Read the model definition and answer for the solid it produces. Units are mm, in the model's axes. A direction names the side the tool comes from. Coordinates: 2 decimals unless noted, no trailing zeros. Write each loop counter-clockwise with the first axis right and the second up, starting at its lowest first coordinate (ties: lowest second). Pieces come first, ordered by that corner, then holes. Notation, with made-up numbers: (76, -26) -> (130, -26) arc R25 ccw to (130, -8) -> close; hole circle Ø9 at (71.25, 61). An arc over 180 degrees is marked (long way). Return JSON: item names as keys, results as strings.
Autodesk Fusion 360 part; units mm, degrees
sketch "Sketch1" plane through (0, 0, 0) normal (0, 1, 0) x (1, 0, 0)
  line L0 (0, 0) -> (41, 0)
  line L1 (41, 0) -> (41, -41)
  line L2 (41, -41) -> (0, -41)
  line L3 (0, -41) -> (0, 0)
  line L4 (0, -20.5) -> (41, -20.5) construction
  line L5 (20.5, 0) -> (20.5, -41) construction
  circle A0 centre (20.5, -20.5) radius 12.5
  line L6 (36, -36) -> (5, -36) construction
  line L7 (5, -36) -> (5, -5) construction
  line L8 (5, -5) -> (36, -5) construction
  line L9 (36, -5) -> (36, -36) construction
  line L10 (36, -36) -> (5, -5) construction
  line L11 (5, -36) -> (36, -5) construction
  circle A1 centre (5, -36) radius 1.8
  circle A2 centre (36, -36) radius 1.8
  circle A3 centre (36, -5) radius 1.8
  circle A4 centre (5, -5) radius 1.8
  circle A5 centre (5, -36) radius 3.25
  circle A6 centre (36, -36) radius 3.25
  circle A7 centre (36, -5) radius 3.25
  circle A8 centre (5, -5) radius 3.25
  line L12 (0, -10.5) -> (13, -10.5)
  line L13 (13, -30.5) -> (0, -30.5)
  point P0 (20.5, -20.5)
  dimension "d1" = 31
  dimension "d2" = 31
  dimension "d3" = 25
  dimension "d4" = 3.6
  dimension "d5" = 3.6
  dimension "d6" = 3.6
  dimension "d7" = 3.6
  dimension "d8" = 6.5
  dimension "d9" = 6.5
  dimension "d10" = 6.5
  dimension "d11" = 6.5
  dimension "d12" = 41
  dimension "d13" = 10
  dimension "d14" = 10
extrude "Extrude1" add sketch "Sketch1" along normal blind 2 contours L0 L1 L2 L3 A0 L12 L13 | A5 | A6 | A7 | A8
extrude "Extrude2" add sketch "Sketch1" along normal blind 30.7 contours A5 | A6 | A7 | A8
ref_plane "WorkPlane1" through (20.5, 1, 20.5) normal (0, 0, 1) x (1, 0, 0)
fillet "Fillet1" radius 1 4 edges at (32.9699, 2, 34.8247) (32.9699, 2, 3.8247) (1.9699, 2, 3.8247) (1.9699, 2, 34.8247)
fillet "Fillet2" radius 4.5 6 edges at (41, 1, 0) (41, 1, 41) (0, 1, 0) (0, 1, 41) (0, 1, 10.5) (0, 1, 30.5)
equation "d2 = d1"
equation "d5 = d4"
equation "d6 = d5"
equation "d7 = d4"
equation "d9 = d8"
equation "d10 = d8"
equation "d11 = d8"
equation "d14 = d13"
equation "Hoogte = 30.7 mm"
equation "d18 = Hoogte"
equation "d20 = ( -41 / 2 ) * 1 mm"
1. The part is cut by section C-C (x = 20.5). Determine the outline of the cut face in (y, z), then the cut area to 3 significant figures.
Taken from the geometry:
{"outline": "(0, 0) -> (2, 0) -> (2, 8) -> (0, 8) -> close; (0, 33) -> (2, 33) -> (2, 41) -> (0, 41) -> close", "area": "32.0 mm2"}
2. The part is cut by section D-D (z = 20.5). Determine the outline of the cut face in (x, y).
Taken from the geometry:
{"outline": "(33, 0) -> (41, 0) -> (41, 2) -> (33, 2) -> close"}
3. A tool of negligible diameter and unlimited length cuts with its end or side. For faces 5 (the face through (1.283, 1.014, 9.147)), 6 (the face through (8.1, 16.66, 5.98)), 7 (the face through (0, 1, 36)), from which of +Z, -Z, +X, -X, +Y, -Y can it reach the whole face along a straight path? Write none if from no direction.
Taken from the geometry:
{"face 5": "-X, +Y, -Y", "face 6": "+Y", "face 7": "+Z, -Z, -X, +Y, -Y"}
4. Consider L1, parallel to Z at x = 5, y = 7; L2, parallel to Z at x = 4, y = 4. Determine where each line is inside the solid, lowest interval first.
Taken from the geometry:
{"L1": "z = 1.75 to 3.2, 6.8 to 8.25, 32.75 to 34.2, 37.8 to 39.25", "L2": "z = 1.91 to 3.5, 6.5 to 8.09, 32.91 to 34.5, 37.5 to 39.09"}
5. The part is cut by section B-B (x = 10.5). Determine the outline of the cut face in (y, z), then the cut area to 3 significant figures.
Taken from the geometry:
{"outline": "(0, 0) -> (2, 0) -> (2, 10.5) -> (0, 10.5) -> close; (0, 30.5) -> (2, 30.5) -> (2, 41) -> (0, 41) -> close", "area": "42.0 mm2"}
6. For a pull along X with two mould halves and no side action, classify faces 1 (the face through (37.717, 15.135, 36.541)), 2 (the face through (39.647, 1.014, 39.717)), 3 (the face through (9, 1, 10.5)), 4 (the face through (4.295, 16.656, 32.827)) as +X half, -X half, draft (parallel to the pull), parting line (faces both ways), or undercut.
Taken from the geometry:
{"face 1": "undercut", "face 2": "+X half", "face 3": "draft", "face 4": "undercut"}
7. Flat-ended cylindrical pins translate along their axes: pin 1 Ø3 at (x, z) = (5, 5) entering from -Y; pin 2 Ø3 at (y, z) = (18, 9) entering from +X; pin 3 Ø8 at (y, z) = (18.5, 30) entering from +X; pin 4 Ø12.5 at (x, z) = (29.5, 17) entering from +Y. Find the tip coordinate at first contact, or state that the pin passes through.
Taken from the geometry:
{"pin 1": "passes through", "pin 2": "stops at x = 38.08", "pin 3": "stops at x = 38.56", "pin 4": "stops at y = 2"}
8. The part is cut by section A-A (y = 17). Determine the outline of the cut face in (x, z), then the cut area to 3 significant figures.
Taken from the geometry:
{"outline": "circle Ø6.5 at (5, 5); circle Ø6.5 at (5, 36); circle Ø6.5 at (36, 5); circle Ø6.5 at (36, 36); hole circle Ø3.6 at (5, 5); hole circle Ø3.6 at (5, 36); hole circle Ø3.6 at (36, 5); hole circle Ø3.6 at (36, 36)", "area": "92.0 mm2"}
